Geometry: final body of the model. Coordinates: model frame, mm. Round coordinates to 2 decimals unless told otherwise and drop trailing zeros. Loops run counter-clockwise (first coordinate to the right, second up) from the corner with the lowest first, then second, coordinate; pieces in that order, holes last. Notation, with made-up numbers: M 14,63.25 L 43,63.25 A17 ccw 43,95.25 Z; hole C 17.5,1 d11. An arc over 180 degrees is marked long. Write each question's results on one line, items separated by ' | '.
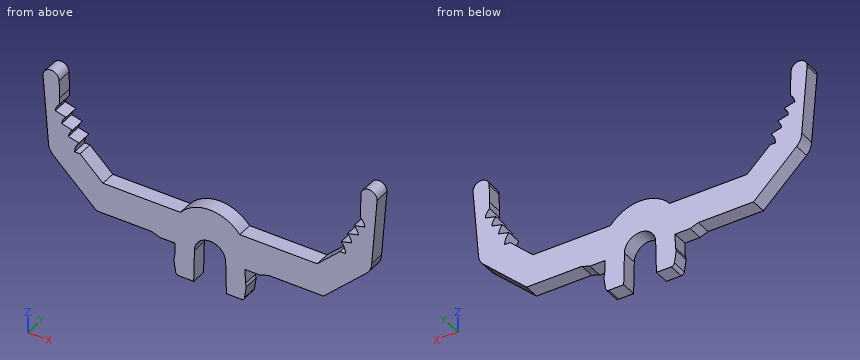
```python
from build123d import *

# Parameters (mm, degrees)
F1_DEPTH = 2.85


with BuildPart() as f1:
    # F0 (on Front) → F1 (new body)
    with BuildSketch(Plane.XZ):
        with BuildLine():
            Line((-5.5, 25.817474), (-19.875, 25.817474))
            Line((-19.875, 25.817474), (-24.125, 29.817474))
            Line((-24.125, 29.817474), (-25.125, 29.817474))
            ThreePointArc((-25.125, 29.817474), (-24.917582, 30.894507), (-24.325, 31.817474))
            Line((-24.325, 31.817474), (-26.281571, 32.317474))
            ThreePointArc((-26.281571, 32.317474), (-26.014286, 33.123461), (-25.525, 33.817474))
            Line((-25.525, 33.817474), (-27.524757, 34.317474))
            ThreePointArc((-27.524757, 34.317474), (-27.269126, 35.144383), (-26.725, 35.817474))
            Line((-26.725, 35.817474), (-28.724757, 36.317474))
            ThreePointArc((-28.724757, 36.317474), (-28.469126, 37.144383), (-27.925, 37.817474))
            Line((-27.925, 37.817474), (-27.925, 39.067474))
            Line((-27.925, 39.067474), (-28.000395, 42.351898))
            ThreePointArc((-28.000395, 42.351898), (-29.517213, 43.817376), (-31, 42.317474))
            Line((-31, 42.317474), (-30.000272, 29.777114))
            ThreePointArc((-30.000272, 29.777114), (-29.754203, 28.587215), (-29.056366, 27.592514))
            Line((-29.056366, 27.592514), (-21.061011, 20.067474))
            Line((-21.061011, 20.067474), (-10.8, 20.067474))
            Line((-10.8, 20.067474), (-9.3, 19.517474))
            Line((-9.3, 19.517474), (-6.49904, 19.517474))
            Line((-6.49904, 19.517474), (-6.560163, 16.867474))
            Line((-6.560163, 16.867474), (-6.725, 16.267474))
            Line((-6.725, 16.267474), (-6.378565, 14.025835))
            ThreePointArc((-6.378565, 14.025835), (-6.176127, 13.661962), (-5.785604, 13.517474))
            Line((-5.785604, 13.517474), (-3.037433, 13.517474))
            Line((-3.037433, 13.517474), (-2.89904, 19.517474))
            ThreePointArc((-2.89904, 19.517474), (0, 22.416514), (2.89904, 19.517474))
            Line((2.89904, 19.517474), (3.037433, 13.517474))
            Line((3.037433, 13.517474), (5.785604, 13.517474))
            ThreePointArc((5.785604, 13.517474), (6.176127, 13.661962), (6.378565, 14.025835))
            Line((6.378565, 14.025835), (6.725, 16.267474))
            Line((6.725, 16.267474), (6.560163, 16.867474))
            Line((6.560163, 16.867474), (6.49904, 19.517474))
            Line((6.49904, 19.517474), (9.3, 19.517474))
            Line((9.3, 19.517474), (10.8, 20.067474))
            Line((10.8, 20.067474), (21.061011, 20.067474))
            Line((21.061011, 20.067474), (29.056366, 27.592514))
            ThreePointArc((29.056366, 27.592514), (29.754203, 28.587215), (30.000272, 29.777114))
            Line((30.000272, 29.777114), (31, 42.317474))
            ThreePointArc((31, 42.317474), (29.517213, 43.817376), (28.000395, 42.351898))
            Line((28.000395, 42.351898), (27.925, 39.067474))
            Line((27.925, 39.067474), (27.925, 37.817474))
            ThreePointArc((27.925, 37.817474), (28.469126, 37.144383), (28.724757, 36.317474))
            Line((28.724757, 36.317474), (26.725, 35.817474))
            ThreePointArc((26.725, 35.817474), (27.269126, 35.144383), (27.524757, 34.317474))
            Line((27.524757, 34.317474), (25.525, 33.817474))
            ThreePointArc((25.525, 33.817474), (26.014286, 33.123461), (26.281571, 32.317474))
            Line((26.281571, 32.317474), (24.325, 31.817474))
            ThreePointArc((24.325, 31.817474), (24.917582, 30.894507), (25.125, 29.817474))
            Line((25.125, 29.817474), (24.125, 29.817474))
            Line((24.125, 29.817474), (19.875, 25.817474))
            Line((19.875, 25.817474), (5.5, 25.817474))
            ThreePointArc((5.5, 25.817474), (0, 28.416514), (-5.5, 25.817474))
        make_face()
    extrude(amount=F1_DEPTH)


solid = f1.part
```
1. Section B-B (x = -22). Output: boundary loops of the cut face in (y, z), then the cut area to 3 significant figures.
Answer key:
outline: M -2.85,20.95 L 0,20.95 L 0,27.82 L -2.85,27.82 Z | area: 19.6 mm²
2. Section A-A (x = 0). Output: boundary loops of the cut face in (y, z), then the cut area to 3 significant figures.
Answer key:
outline: M -2.85,22.42 L 0,22.42 L 0,28.42 L -2.85,28.42 Z | area: 17.1 mm²
3. Pin query (flat end, axial travel): P1, Ø0.5, axis at x = 24.5, y = -1.5, coming from the +Z side; P2, Ø1.4, axis at x = 13, y = -2, coming from the +Z side; P3, Ø0.9, axis at x = 18, y = -2, coming from the -Z side; P4, Ø1.5, axis at x = -16, z = 18, coming from the -Y side. Return the tip coordinate at first contact, or that it passes through.
Answer key:
P1: stops at z = 31.93 | P2: stops at z = 25.82 | P3: stops at z = 20.07 | P4: passes through
4. Ray query, probe 1 along Z at (x, y) = (13, -1.9); probe 2 along Z at (x, y) = (24.5, -2); probe 3 along X at (y, z) = (-0.7, 42). Return the intervals inside material, ascending.
Answer key:
probe 1: z = 20.07 to 25.82 | probe 2: z = 23.3 to 29.82, 31.62 to 31.86 | probe 3: x = -30.97 to -27.99, 27.99 to 30.97
